from build123d import *

# Parameters (mm, degrees)
SKETCH1_W           = 57
SKETCH1_H           = 57
SKETCH1_R           = 2.5
BOSS_EXTRUDE2_DEPTH = 99
SKETCH3_W           = 10
SKETCH3_H           = 10
CUT_EXTRUDE1_DEPTH  = 89
CHAMFER1_SIZE       = 3
SKETCH4_R           = 19.05
BOSS_EXTRUDE5_DEPTH = 1.6
SKETCH9_R           = 4.025639025
CUT_EXTRUDE3_DEPTH  = 1.6


with BuildPart() as part:
    # Sketch1 → Boss-Extrude2 (new body)
    with BuildSketch(Plane.XY):
        Rectangle(SKETCH1_W, SKETCH1_H)
        with Locations((23.55, -23.55)):
            Circle(SKETCH1_R, mode=Mode.SUBTRACT)
        with Locations((23.55, 23.55)):
            Circle(SKETCH1_R, mode=Mode.SUBTRACT)
        with Locations((-23.55, 23.55)):
            Circle(SKETCH1_R, mode=Mode.SUBTRACT)
        with Locations((-23.55, -23.55)):
            Circle(SKETCH1_R, mode=Mode.SUBTRACT)
    extrude(amount=BOSS_EXTRUDE2_DEPTH)

    # Sketch3 → Cut-Extrude1 (cut)
    with BuildSketch(Plane.XY.offset(99)):
        with Locations((-23.5, 23.5)):
            Rectangle(SKETCH3_W, SKETCH3_H)
        with Locations((-23.5, -23.5)):
            Rectangle(SKETCH3_W, SKETCH3_H)
        with Locations((23.5, -23.5)):
            Rectangle(SKETCH3_W, SKETCH3_H)
        with Locations((23.5, 23.5)):
            Rectangle(SKETCH3_W, SKETCH3_H)
    extrude(amount=-CUT_EXTRUDE1_DEPTH, mode=Mode.SUBTRACT)

    # Chamfer1
    chamfer1_edges = [part.edges().sort_by_distance(p)[0] for p in [
        (-18.5, -18.5, 54.5),
        (18.5, -18.5, 54.5),
        (18.5, 18.5, 54.5),
        (-18.5, 18.5, 54.5),
    ]]
    chamfer(chamfer1_edges, length=CHAMFER1_SIZE)

    # Sketch4 → Boss-Extrude5 (add)
    with BuildSketch(Plane(origin=(0, 0, 0), x_dir=(-1, 0, 0), z_dir=(0, 0, -1))):
        Circle(SKETCH4_R)
    extrude(amount=BOSS_EXTRUDE5_DEPTH)

    # Sketch9 → Cut-Extrude3 (cut)
    with BuildSketch(Plane(origin=(0, 0, -1.6), x_dir=(-1, 0, 0), z_dir=(0, 0, -1))):
        Circle(SKETCH9_R)
    extrude(amount=-CUT_EXTRUDE3_DEPTH, mode=Mode.SUBTRACT)


solid = part.part
Can you work these out from the model? Positions are in its coordinate system, mm. A direction names the side the tool comes from. Coordinates: 2 decimals unless noted, no trailing zeros. Order: outer loops, then holes, each group sorted by start corner. A loop starts at its lowest first (then second) coordinate and runs counter-clockwise, first axis right, second up. Notation, with made-up numbers: (-21, -30) -> (18, -30) arc R23 ccw to (18, -9) -> close; hole circle Ø7 at (-14.5, -14). An arc over 180 degrees is marked (long way). Use one line per item in the form item = value.
Q1. I need wall thicknesses on L1, parallel to Y at x = -23.55, z = 2.5; L2, parallel to Z at x = 24, y = 7. Which ranges of each line are inside material? Lowest first, please.
From the geometry:
L1 = -28.5 to -26.05, -21.05 to 21.05, 26.05 to 28.5
L2 = 0 to 99
Q2. Which directions (+Z, -Z, +X, -X, +Y, -Y) give clear straight access to the entire face, cutting with the end or side of a thin tool? Please do faces 1 (the face through (25, 18.5, 55)), 2 (the face through (-26, 25, 10)), 3 (the face through (15.12, -11.59, -0.79)).
From the geometry:
face_1 = +Z, +X, +Y
face_2 = +Z, -X, +Y
face_3 = -Z
Q3. Will these pins go through, and if not, where does the flat tip stop? P1, Ø5, axis at x = 23, y = -23.5, coming from the +Z side; P2, Ø2, axis at y = 26.5, z = 48, coming from the +X side; P3, Ø7.5, axis at x = 24.5, z = 71, coming from the +Y side; P4, Ø4.5, axis at x = 23.55, y = 23.55, coming from the +Z side.
From the geometry:
P1 = 10
P2 = 18.5
P3 = 19.25
P4 = through
Q4. We'd pull the mould along X, two halves only. Please class faces 4 (the face through (-20, -20, 55)), 5 (the face through (23.01, -25.99, 4.93)), 6 (the face through (0, 0, 99)): released by +X, released by -X, zero draft, split by the parting line, or undercut.
From the geometry:
face_4 = released by -X
face_5 = undercut
face_6 = zero draft
Q5. Imagine slicing it at A-A, the plane x = -23.55. List the corners of the cut face in (y, z) for me, then the cut area to 3 significant figures.
From the geometry:
outline = (-28.5, 0) -> (-26.05, 0) -> (-26.05, 10) -> (-28.5, 10) -> close; (-21.05, 0) -> (21.05, 0) -> (21.05, 10) -> (18.5, 10) -> (18.5, 99) -> (-18.5, 99) -> (-18.5, 10) -> (-21.05, 10) -> close; (26.05, 0) -> (28.5, 0) -> (28.5, 10) -> (26.05, 10) -> close
area = 3,760 mm²
Q6. Imagine slicing it at D-D, the plane z = 87. List the corners of the cut face in (x, y) for me.
From the geometry:
outline = (-28.5, -18.5) -> (-21.5, -18.5) -> (-18.5, -21.5) -> (-18.5, -28.5) -> (18.5, -28.5) -> (18.5, -21.5) -> (21.5, -18.5) -> (28.5, -18.5) -> (28.5, 18.5) -> (21.5, 18.5) -> (18.5, 21.5) -> (18.5, 28.5) -> (-18.5, 28.5) -> (-18.5, 21.5) -> (-21.5, 18.5) -> (-28.5, 18.5) -> close
Q7. Imagine slicing it at C-C, the plane z = 7. List the corners of the cut face in (x, y) for me, then the cut area to 3 significant figures.
From the geometry:
outline = (-28.5, -28.5) -> (28.5, -28.5) -> (28.5, 28.5) -> (-28.5, 28.5) -> close; hole circle Ø5 at (-23.55, -23.55); hole circle Ø5 at (-23.55, 23.55); hole circle Ø5 at (23.55, -23.55); hole circle Ø5 at (23.55, 23.55)
area = 3,170 mm²
